Geometry: see drawing. Coordinates: mm, zero at the bounding-box minimum. A direction names the side the tool comes from. Coordinates: 2 decimals unless noted, no trailing zeros. Write each loop counter-clockwise with the first axis right and the second up, starting at its lowest first coordinate (ties: lowest second). Pieces come first, ordered by that corner, then holes. Notation, with made-up numbers: M 77,79.25 L 90,79.25 A9 cw 90,87.25 Z; hole C -15.5,31 d10. An arc over 180 degrees is marked long. Answer as CSV lines item,"result". Start each with the question number.
1. Section A-A on z = 9. Return the cut outline in (x, y) (3 decimals), plus the area to 3 significant figures.
2. Contact query for flat-ended pins moving along their axis: pin 1 Ø6.5 at (x, z) = (10.075, 9) entering from -Y; pin 2 Ø1.5 at (y, z) = (15, 8.5) entering from +X; pin 3 Ø10 at (y, z) = (9.5, 8) entering from -X. Output: stop coordinate, or through.
3. Line query: probe 1 along Y at (x, z) = (1.25, 9) (3 decimals); probe 2 along Y at (x, z) = (13.75, 3); probe 3 along X at (y, z) = (3, 8.5). Output: solid intervals per line, ascending. Write a range as [from, to].
4. Mould query, pull axis Z, two halves, no side actions, for the marked faces 1 and 2. Classes: pulls with the +Z half, pulls with the -Z half, needs draft (parallel to the pull), parting line crosses it, or undercut.
5. Reachability of the marked faces 3 and 4 from +Z, -Z, +X, -X, +Y, -Y: full face, straight path, thin tool, end or side. Return the list, or none.
6. Section D-D on z = 13.25. Return the cut outline in (x, y).
7. Section C-C on x = 9. Return the cut outline in (y, z).
8. Section B-B on y = 12.5. Return the cut outline in (x, z).
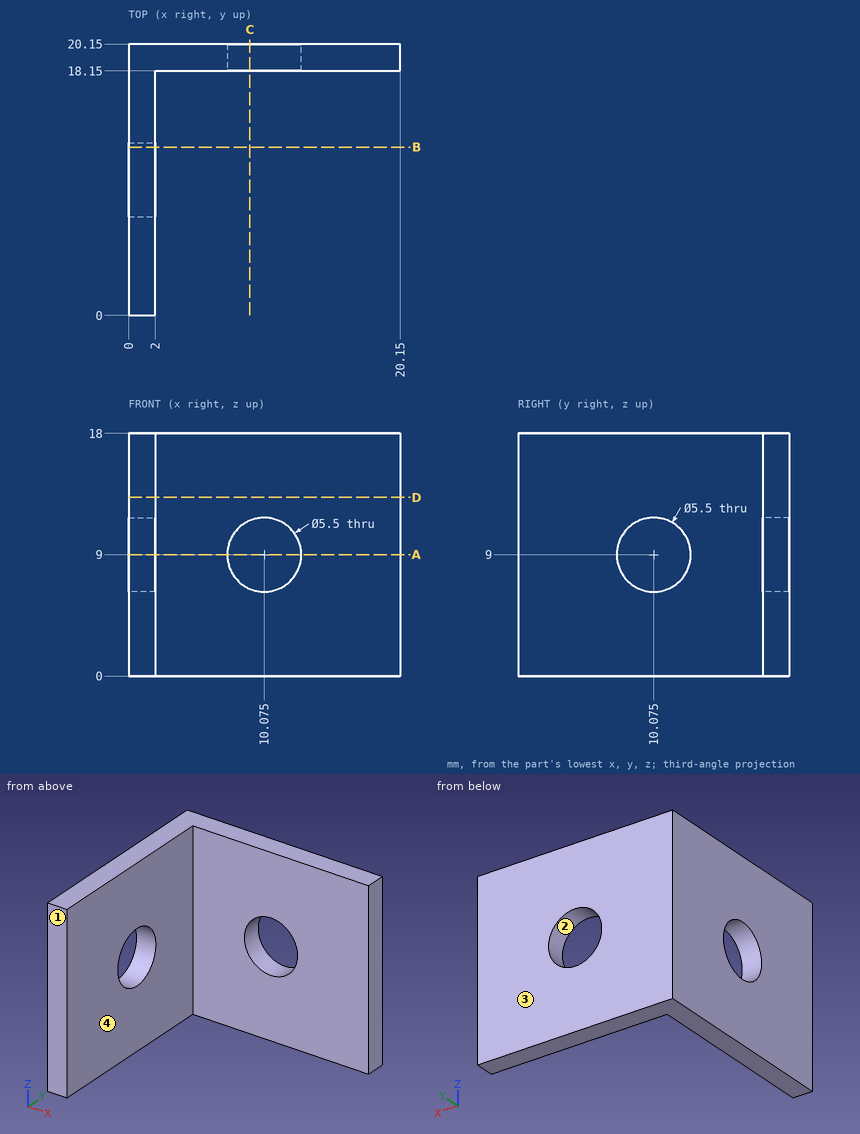
Values:
1,outline,"M 0,0 L 2,0 L 2,7.325 L 0,7.325 Z; M 0,12.825 L 2,12.825 L 2,18.15 L 7.325,18.15 L 7.325,20.15 L 0,20.15 Z; M 12.825,18.15 L 20.15,18.15 L 20.15,20.15 L 12.825,20.15 Z"
1,area,"54.6 mm²"
2,pin 1,"y = 18.15"
2,pin 2,"x = 2"
2,pin 3,"x = 0"
3,probe 1,"[0, 7.325], [12.825, 20.15]"
3,probe 2,"[18.15, 20.15]"
3,probe 3,"[0, 2]"
4,face 1,"needs draft"
4,face 2,"undercut"
5,face 3,"+Z, -Z, +X, -X, +Y"
5,face 4,"+Z, -Z, +X, -Y"
6,outline,"M 0,0 L 2,0 L 2,18.15 L 20.15,18.15 L 20.15,20.15 L 0,20.15 Z"
7,outline,"M 18.15,0 L 20.15,0 L 20.15,6.47 L 18.15,6.47 Z; M 18.15,11.53 L 20.15,11.53 L 20.15,18 L 18.15,18 Z"
8,outline,"M 0,0 L 2,0 L 2,7.7 L 0,7.7 Z; M 0,10.3 L 2,10.3 L 2,18 L 0,18 Z"
